Can you work these out from the model? Positions are in its coordinate system, mm. Face numbers are marked on the shaded views. Coordinates: 2 decimals unless noted, no trailing zeros. Order: outer loops, then holes, each group sorted by start corner. A loop starts at its lowest first (then second) coordinate and runs counter-clockwise, first axis right, second up. Notation, with made-up numbers: (51, 78.25) -> (68, 78.25) arc R17 ccw to (68, 92.25) -> close; hole circle Ø6 at (40, -10). An arc over 180 degrees is marked (long way). Answer in a Markdown table with one row per item.
```python
from build123d import *

# Parameters (mm, degrees)
BOSS_EXTRUDE1_DEPTH = 8


with BuildPart() as part:
    # Sketch1 → Boss-Extrude1 (new body)
    with BuildSketch(Plane.XY):
        with BuildLine():
            Line((11.445, 13.16), (10.555, 13.16))
            ThreePointArc((10.555, 13.16), (10, 12.605), (9.445, 13.16))
            Line((9.445, 13.16), (8.555, 13.16))
            ThreePointArc((8.555, 13.16), (8, 12.605), (7.445, 13.16))
            Line((7.445, 13.16), (6.555, 13.16))
            ThreePointArc((6.555, 13.16), (6, 12.605), (5.445, 13.16))
            Line((5.445, 13.16), (4.555, 13.16))
            ThreePointArc((4.555, 13.16), (4, 12.605), (3.445, 13.16))
            Line((3.445, 13.16), (2.555, 13.16))
            ThreePointArc((2.555, 13.16), (2, 12.605), (1.445, 13.16))
            Line((1.445, 13.16), (0.555, 13.16))
            ThreePointArc((0.555, 13.16), (0.392444264, 12.767555736), (0, 12.605))
            Line((0, 12.605), (0, 0.555))
            ThreePointArc((0, 0.555), (0.392444264, 0.392444264), (0.555, 0))
            Line((0.555, 0), (1.445, 0))
            ThreePointArc((1.445, 0), (2, 0.555), (2.555, 0))
            Line((2.555, 0), (3.445, 0))
            ThreePointArc((3.445, 0), (4, 0.555), (4.555, 0))
            Line((4.555, 0), (5.445, 0))
            ThreePointArc((5.445, 0), (6, 0.555), (6.555, 0))
            Line((6.555, 0), (7.445, 0))
            ThreePointArc((7.445, 0), (8, 0.555), (8.555, 0))
            Line((8.555, 0), (9.445, 0))
            ThreePointArc((9.445, 0), (10, 0.555), (10.555, 0))
            Line((10.555, 0), (11.445, 0))
            ThreePointArc((11.445, 0), (11.607555736, 0.392444264), (12, 0.555))
            Line((12, 0.555), (12, 12.605))
            ThreePointArc((12, 12.605), (11.607555736, 12.767555736), (11.445, 13.16))
        make_face()
    extrude(amount=BOSS_EXTRUDE1_DEPTH)


solid = part.part
```
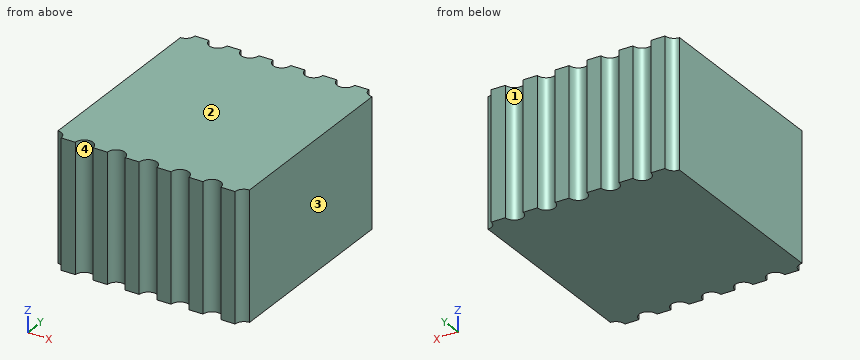
(1) We'd pull the mould along X, two halves only. Please class the marked faces 1, 2, 3 and 4: +X half, -X half, draft (parallel to the pull), parting line (faces both ways), or undercut.
Response values:
| item | result |
|---|---|
| face 1 | undercut |
| face 2 | draft |
| face 3 | +X half |
| face 4 | undercut |
(2) I need wall thicknesses on line 1 (Y direction, x = 10, z = 7) (3 decimals); line 2 (Y direction, x = 1.75, z = 3). Which ranges of each line are inside material? Lowest first, please. Write a range as [from, to].
Response values:
| item | result |
|---|---|
| line 1 | [0.555, 12.605] |
| line 2 | [0.5, 12.66] |
(3) Suppose I cut it at B-B (x = 10). Please give me the cut outline in (y, z) (3 decimals), and give its area (3 significant figures).
Response values:
| item | result |
|---|---|
| outline | (0.555, 0) -> (12.605, 0) -> (12.605, 8) -> (0.555, 8) -> close |
| area | 96.4 mm2 |
(4) Suppose I cut it at A-A (z = 2.5). Please give me the cut outline in (x, y) (3 decimals), and give its area (3 significant figures).
Response values:
| item | result |
|---|---|
| outline | (0, 0.555) arc R0.555 cw to (0.555, 0) -> (1.445, 0) arc R0.555 cw to (2.555, 0) -> (3.445, 0) arc R0.555 cw to (4.555, 0) -> (5.445, 0) arc R0.555 cw to (6.555, 0) -> (7.445, 0) arc R0.555 cw to (8.555, 0) -> (9.445, 0) arc R0.555 cw to (10.555, 0) -> (11.445, 0) arc R0.555 cw to (12, 0.555) -> (12, 12.605) arc R0.555 cw to (11.445, 13.16) -> (10.555, 13.16) arc R0.555 cw to (9.445, 13.16) -> (8.555, 13.16) arc R0.555 cw to (7.445, 13.16) -> (6.555, 13.16) arc R0.555 cw to (5.445, 13.16) -> (4.555, 13.16) arc R0.555 cw to (3.445, 13.16) -> (2.555, 13.16) arc R0.555 cw to (1.445, 13.16) -> (0.555, 13.16) arc R0.555 cw to (0, 12.605) -> close |
| area | 152 mm2 |
